Geometry: see drawing. Coordinates: mm, zero at the bounding-box minimum. Give positions to 0.01 mm unless a question says otherwise; leave off trailing zeros. Write each loop counter-clockwise with the first axis right and the second up, starting at its lowest first coordinate (ties: lowest second). Pieces come first, ordered by that corner, then holes. Notation, with made-up numbers: M 39.5,-37.5 L 83.5,-37.5 A8 ccw 83.5,-27.5 Z; hole C 38,3.5 d11. An arc over 180 degrees is marked long. Use a Markdown table: item, result. Add a question column.
1) Line query: line 1 (Y direction, x = 26.5, z = 3.1); line 2 (Z direction, x = 9, y = 1). Output: solid intervals per line, ascending.
2) Pin query (flat end, axial travel): pin 1 (1 mm diameter, centred on x = 24, z = 5, fed in from -Y). Return the tip coordinate at first contact, or that it passes through.
3) Section A-A on x = 34. Return the cut outline in (y, z), then the cut area to 3 significant figures.
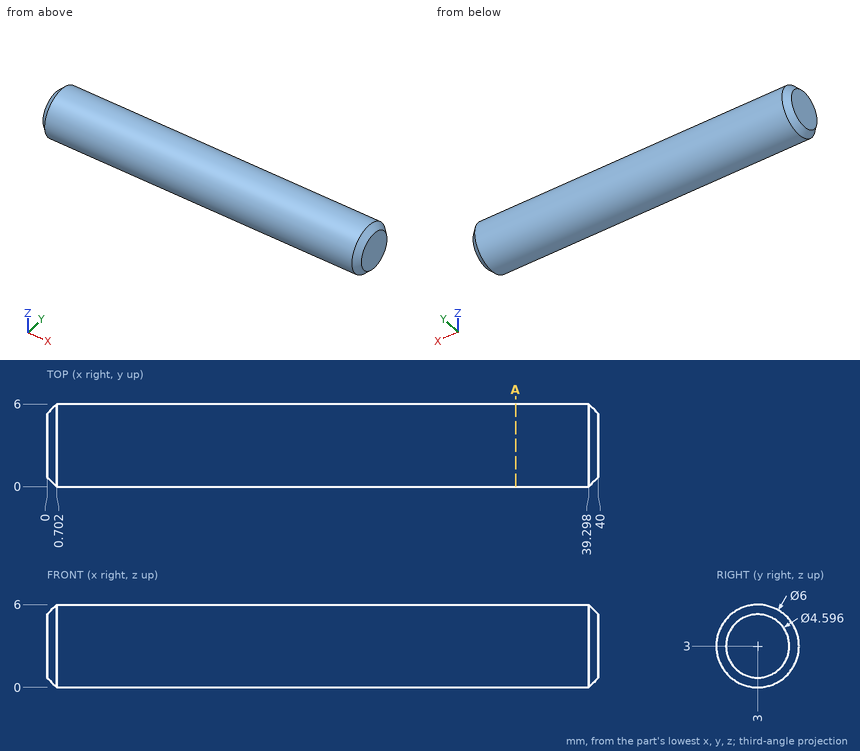
Found:
| question | item | result |
|---|---|---|
| 1 | line 1 | 0 to 6 |
| 1 | line 2 | 0.76 to 5.24 |
| 2 | pin 1 | y = 0.4 |
| 3 | outline | C 3,3 d6 |
| 3 | area | 28.3 mm² |
